```python
from build123d import *

# Parameters (mm, degrees)
SKETCH_1_R      = 3.05
SKETCH_1_R_2    = 5.05
EXTRUDE_1_DEPTH = 4


with BuildPart() as part:
    # 草图1 → 凸台-拉伸1 (new body)
    with BuildSketch(Plane.XY):
        with BuildLine():
            Line((8.424446615, -21.943763958), (1.909734407, -10.659930534))
            ThreePointArc((1.909734407, -10.659930534), (-4.930907825, 4.188585667), (-11.771663917, -10.659878079))
            Line((-11.771663917, -10.659878079), (-18.286394211, -21.943701062))
            ThreePointArc((-18.286394211, -21.943701062), (-23.683045573, -22.611553889), (-27.70998166, -26.265819763))
            Line((-27.70998166, -26.265819763), (-27.725209001, -26.292194242))
            ThreePointArc((-27.725209001, -26.292194242), (-28.893024381, -31.617931514), (-26.77174103, -36.640622744))
            ThreePointArc((-26.77174103, -36.640622744), (-18.28646206, -39.640629543), (-11.445740476, -33.792165797))
            Line((-11.445740476, -33.792165797), (1.583702026, -33.792176239))
            ThreePointArc((1.583702026, -33.792176239), (4.862729341, -38.133535764), (10.044259423, -39.792200488))
            Line((10.044259423, -39.792200488), (10.069016027, -39.792200488))
            ThreePointArc((10.069016027, -39.792200488), (15.265142091, -38.140688354), (18.55427588, -33.792261359))
            ThreePointArc((18.55427588, -33.792261359), (16.909732497, -24.943778842), (8.424446615, -21.943763958))
        make_face()
        with Locations((10.069016027, -30.792200488)):
            Circle(SKETCH_1_R, mode=Mode.SUBTRACT)
        with Locations((-4.930942332, -4.811414333)):
            Circle(SKETCH_1_R_2, mode=Mode.SUBTRACT)
        with Locations((-19.930983973, -30.792200488)):
            Circle(SKETCH_1_R, mode=Mode.SUBTRACT)
        with BuildLine():
            Line((-3.286438615, -13.659894854), (3.228291788, -24.943759794))
            ThreePointArc((3.228291788, -24.943759794), (2.274792619, -26.292204621), (1.583743226, -27.792176239))
            Line((1.583743226, -27.792176239), (-11.445735667, -27.792165797))
            ThreePointArc((-11.445735667, -27.792165797), (-12.136773559, -26.29218888), (-13.090262388, -24.943736742))
            Line((-13.090262388, -24.943736742), (-6.575513898, -13.659882243))
            ThreePointArc((-6.575513898, -13.659882243), (-4.930976838, -13.811414333), (-3.286438615, -13.659894854))
        make_face(mode=Mode.SUBTRACT)
    extrude(amount=EXTRUDE_1_DEPTH)


solid = part.part
```
Model file for the job. Use its own axes, mm. A direction names the side the tool comes from. Coordinates: 2 decimals unless noted, no trailing zeros. Order: outer loops, then holes, each group sorted by start corner. A loop starts at its lowest first (then second) coordinate and runs counter-clockwise, first axis right, second up. Notation, with made-up numbers: (-18.5, 20) -> (-2.5, 20) arc R14 ccw to (-2.5, 47) -> close; hole circle Ø10 at (69.25, 24.25). An arc over 180 degrees is marked (long way). Answer as a JSON object with one key per item and string values. Group by question number.
1) Cut at A-A, the plane y = -23. Write the cut outline in (x, z).
2) Flat gauge pins, fed straight in: pin 1 (2 mm diameter, centred on x = -2, z = 1, fed in from -Y); pin 2 (2 mm diameter, centred on x = -9.5, y = -35, fed in from -Z); pin 3 (2 mm diameter, centred on y = -26.5, z = 1, fed in from -X). Where does each tip first touch, or does it go through?
3) Which spindle directions (+Z, -Z, +X, -X, +Y, -Y) get a long thin tool onto all of the face, cutting with end or side? Do faces 4 (the face through (-0.075, -19.223, 1.972)), 5 (the face through (0, -17, 0)), 6 (the face through (4.8, -38.09, 1.97)). Say none if no direction does.
4) Cut at B-B, the plane x = 12.5. Write the cut outline in (y, z), then the cut area to 3 significant figures.
5) Drill centre lines: L1, parallel to X at y = -31, z = 3.75; L2, parallel to Y at x = -12, z = 2.7; L3, parallel to Y at x = -7, z = 1.9. Where is each one in solid material? Low to high.
6) Cut at D-D, the plane z = 1.1. Count the separate pieces of the cut face and the enclosed holes in it, then the cut area to 3 significant figures.
7) Cut at C-C, the plane x = -4.5. Write the cut outline in (y, z).
8) Pull direction X, two halves, no side cores. Call faces 1 (the face through (-5, -33.792, 2)), 2 (the face through (0, -17, 4)), 3 (the face through (-4.644, 4.184, 1.972)): +X half, -X half, draft (parallel to the pull), parting line (faces both ways), or undercut.
Check values:
{
 "1": {"outline": "(-24.43, 0) -> (-11.97, 0) -> (-11.97, 4) -> (-24.43, 4) -> close; (2.11, 0) -> (14.57, 0) -> (14.57, 4) -> (2.11, 4) -> close"},
 "2": {"pin 1": "stops at y = -33.79", "pin 2": "passes through", "pin 3": "stops at x = -28.31"},
 "3": {"face 4": "+Z, -Z", "face 5": "-Z, +X, -X, +Y, -Y", "face 6": "+Z, -Z, -Y"},
 "4": {"outline": "(-39.46, 0) -> (-32.63, 0) -> (-32.63, 4) -> (-39.46, 4) -> close; (-28.95, 0) -> (-22.13, 0) -> (-22.13, 4) -> (-28.95, 4) -> close", "area": "54.6 mm²"},
 "5": {"L1": "x = -28.93 to -22.97, -16.89 to 7.03, 13.11 to 19.07", "L2": "y = -35.05 to -26.54, -23.06 to -11.06, -10.38 to 0.76", "L3": "y = -33.79 to -27.79, -14.4 to -9.42, -0.2 to 3.95"},
 "6": {"separate pieces": "1", "enclosed holes": "4", "area": "847 mm²"},
 "7": {"outline": "(-33.79, 0) -> (-27.79, 0) -> (-27.79, 4) -> (-33.79, 4) -> close; (-13.8, 0) -> (-9.84, 0) -> (-9.84, 4) -> (-13.8, 4) -> close; (0.22, 0) -> (4.18, 0) -> (4.18, 4) -> (0.22, 4) -> close"},
 "8": {"face 1": "undercut", "face 2": "draft", "face 3": "parting line"}
}
